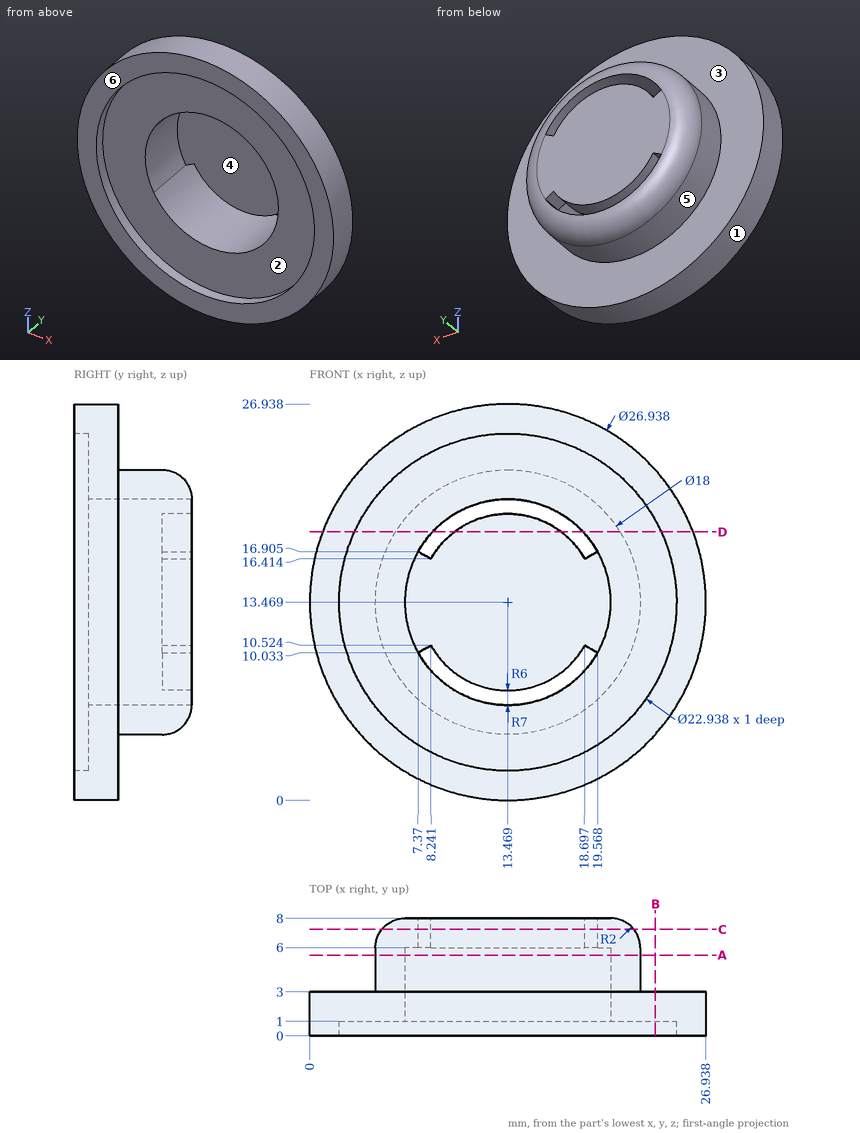
Could you check a few things on this drawing? It's one solid part, dimensions in mm from its lowest x, y, z. A direction names the side the tool comes from. Coordinates: 2 decimals unless noted, no trailing zeros. Order: outer loops, then holes, each group sorted by start corner. A loop starts at its lowest first (then second) coordinate and runs counter-clockwise, first axis right, second up. Notation, with made-up numbers: M 70.25,-7 L 75.25,-7 A18 ccw 75.25,10 Z; hole C 57.5,17 d6. An arc over 180 degrees is marked long. Answer as a JSON object with one key per item and string values. Group by question number.
(1) I need wall thicknesses on probe 1 along Z at (x, y) = (15, 2.75); probe 2 along X at (y, z) = (5.5, 15.5); probe 3 along Z at (x, y) = (10.75, 4). Which ranges of each line are inside material? Lowest first, please.
(2) Which directions (+Z, -Z, +X, -X, +Y, -Y) give clear straight access to the entire face, cutting with the end or side of a thin tool? Please do the marked faces 1, 2 and 3.
(3) Suppose I cut it at D-D, the plane z = 18.25. State how many separate pieces and enclosed holes the cut face has.
(4) Suppose I cut it at A-A, the plane y = 5.5. Please give me the cut outline in (x, z) (1 decimal).
(5) If we mould it in two halves opening along X, with no side actions, what happens to the marked faces 4, 5 and 6? For each: released by +X, released by -X, zero draft, split by the parting line, or undercut.
(6) Suppose I cut it at C-C, the plane y = 7.25. Please give me the cut outline in (x, z) (1 decimal), then the cut area to 3 significant figures.
(7) Suppose I cut it at B-B, the plane x = 23.5. Please give me the cut outline in (y, z), then the cut area to 3 significant figures.
(8) For pin 1 (1.5 mm diameter, centred on x = 5, z = 19.5, fed in from -Y); pin 2 (2 mm diameter, centred on x = 7, y = 1.5, fed in from +Z); pin 3 (2 mm diameter, centred on y = 6.5, z = 13.5, fed in from -X), each with a flat end and sliding along its axis, tell me the tip position at first contact or that it passes through.
Values found:
{
 "1": {"probe 1": "z = 0.09 to 6.64, 20.3 to 26.85", "probe 2": "x = 4.7 to 6.77, 20.17 to 22.24", "probe 3": "z = 4.89 to 7.02, 19.92 to 22.05"},
 "2": {"face 1": "+Y, -Y", "face 2": "-Y", "face 3": "+Y"},
 "3": {"separate pieces": "3", "enclosed holes": "0"},
 "4": {"outline": "C 13.5,13.5 d18; hole C 13.5,13.5 d14"},
 "5": {"face 4": "undercut", "face 5": "split by the parting line", "face 6": "zero draft"},
 "6": {"outline": "C 13.5,13.5 d17.1; hole M 7.4,10 A7 ccw 19.6,10 L 18.7,10.5 A6 cw 8.2,10.5 Z; hole M 7.4,16.9 L 8.2,16.4 A6 cw 18.7,16.4 L 19.6,16.9 A7 ccw Z", "area": "203 mm^2"},
 "7": {"outline": "M 0,4.48 L 3,4.48 L 3,22.46 L 0,22.46 L 0,19.03 L 1,19.03 L 1,7.91 L 0,7.91 Z", "area": "42.8 mm^2"},
 "8": {"pin 1": "stops at y = 1", "pin 2": "stops at z = 25.78", "pin 3": "stops at x = 4.47"}
}
